Could you check a few things on this model? Use its own coordinates, in mm. Give positions to 0.01 mm unless a question says otherwise; leave off trailing zeros. Write each loop counter-clockwise with the first axis right and the second up, starting at its lowest first coordinate (ties: lowest second). Pieces come first, ordered by that corner, then holes. Notation, with made-up numbers: (9, 55) - (43, 55) arc R30 cw to (43, 94) - close; hole circle Ø6 at (21.25, 28.5). An arc over 180 degrees is marked (long way). Use one line per item in the form item = value.
```python
from build123d import *

# Parameters (mm, degrees)
SKETCH093_W      = 26
SKETCH093_H      = 70
EXTRUDE081_DEPTH = 1
SKETCH_W         = 45
SKETCH_H         = 66
EXTRUDE_DEPTH    = 2


with BuildPart() as extrude081:
    # Sketch093 → Extrude081 (new body, symmetric)
    with BuildSketch(Plane.XY.offset(-22)):
        with Locations((62, 50)):
            Rectangle(SKETCH093_W, SKETCH093_H)
    extrude(amount=EXTRUDE081_DEPTH, both=True)


with BuildPart() as cut012:
    # Sketch → Extrude (new body)
    with BuildSketch(Plane(origin=(0, 0, -22), x_dir=(1, 0, 0), z_dir=(0, 0, -1))):
        Polygon((-7, 2), (81, 2), (81, -102), (-7, -102), (-7, -100), (-2, -100), (-2, -93.5), (-4, -93.5), (-4, -9), (-2, -9), (-2, 0), (-7, 0), align=None)
        with Locations((20.5, -52)):
            Rectangle(SKETCH_W, SKETCH_H, mode=Mode.SUBTRACT)
    extrude(amount=EXTRUDE_DEPTH)

    # Cut012: cut Extrude081
    add(extrude081.part, mode=Mode.SUBTRACT)


solid = cut012.part
```
1. For pin 1 (1.1 mm diameter, centred on y = 42.5, z = -22.5, fed in from -X), with a flat end and sliding along its axis, tell me the tip position at first contact or that it passes through.
Response values:
pin_1 = -4
2. If we mould it in two halves opening along Y, with no side actions, what happens to faces 1 (the face through (47, 38, -22)), 2 (the face through (62, 50, -23))? For each: pulls with the +Y half, pulls with the -Y half, needs draft (parallel to the pull), parting line crosses it, or undercut.
Response values:
face_1 = needs draft
face_2 = undercut
3. Imagine slicing it at A-A, the plane y = 34. List the corners of the cut face in (x, z) for me.
Response values:
outline = (-4, -24) - (-2, -24) - (-2, -22) - (-4, -22) - close; (43, -24) - (81, -24) - (81, -22) - (75, -22) - (75, -23) - (49, -23) - (49, -22) - (43, -22) - close
4. Imagine slicing it at D-D, the plane x = 65. List the corners of the cut face in (y, z) for me, and give its area (3 significant figures).
Response values:
outline = (-2, -24) - (102, -24) - (102, -22) - (85, -22) - (85, -23) - (15, -23) - (15, -22) - (-2, -22) - close
area = 138 mm²
5. If I drill on line 1 (X direction, y = 37, z = -22.45); line 2 (Y direction, x = 29.5, z = -22.65); line 3 (X direction, y = 83.5, z = -23.75), over which ranges is the centre line in solid material (lowest first)? Write a range as from..to.
Response values:
line_1 = -4..-2, 43..49, 75..81
line_2 = -2..19, 85..102
line_3 = -4..-2, 43..81
6. Imagine slicing it at C-C, the plane z = -22.3. List the corners of the cut face in (x, y) for me.
Response values:
outline = (-7, -2) - (81, -2) - (81, 102) - (-7, 102) - (-7, 100) - (-2, 100) - (-2, 93.5) - (-4, 93.5) - (-4, 9) - (-2, 9) - (-2, 0) - (-7, 0) - close; hole (-2, 19) - (43, 19) - (43, 85) - (-2, 85) - close; hole (49, 15) - (75, 15) - (75, 85) - (49, 85) - close
7. Imagine slicing it at B-B, the plane x = 25. List the corners of the cut face in (y, z) for me.
Response values:
outline = (-2, -24) - (19, -24) - (19, -22) - (-2, -22) - close; (85, -24) - (102, -24) - (102, -22) - (85, -22) - close
